Here's how the part is built. I have some questions about the finished solid (model axes, mm). A direction names the side the tool comes from. Round coordinates to 2 decimals unless told otherwise and drop trailing zeros. Loops run counter-clockwise (first coordinate to the right, second up) from the corner with the lowest first, then second, coordinate; pieces in that order, holes last. Notation, with made-up numbers: (43, 44) -> (94, 44) arc R30 ccw to (94, 66) -> close; hole circle Ø5 at (-29, 68). An arc over 180 degrees is marked (long way). Use CSV: the item, a comma, the result in double quotes. Start each with the question number.
from build123d import *

# Parameters (mm, degrees)
ESTRUSIONE_ESTRUSIONE1_DEPTH           = 5
SCHIZZO2_W                             = 20
SCHIZZO2_H                             = 6
TAGLIO_ESTRUSIONE1_DEPTH               = 4
FORO_SVASATO_PER_VITE_M2_1_D           = 2.4
FORO_SVASATO_PER_VITE_M2_1_DEPTH       = 4
FORO_SVASATO_PER_VITE_M2_1_CSINK_D     = 4.4
FORO_SVASATO_PER_VITE_M2_1_CSINK_ANGLE = 90
SCHIZZO6_R                             = 2
TAGLIO_ESTRUSIONE3_DEPTH               = 38
SCHIZZO8_R                             = 3
TAGLIO_ESTRUSIONE4_DEPTH               = 3
FORO_SVASATO_PER_VITE_M2_2_D           = 2.4
FORO_SVASATO_PER_VITE_M2_2_DEPTH       = 4
FORO_SVASATO_PER_VITE_M2_2_CSINK_D     = 4.4
FORO_SVASATO_PER_VITE_M2_2_CSINK_ANGLE = 90


with BuildPart() as part:
    # Schizzo1 → Estrusione-Estrusione1 (new body)
    with BuildSketch(Plane(origin=(0, 0, 0), x_dir=(1, 0, 0), z_dir=(0, 1, 0))):
        with BuildLine():
            Line((-29.167003354, 45), (90.832996646, 45))
            Line((90.832996646, 45), (110.832996646, 25))
            Line((110.832996646, 25), (110.832996646, -25))
            Line((110.832996646, -25), (90.832996646, -45))
            Line((90.832996646, -45), (-29.167003354, -45))
            ThreePointArc((-29.167003354, -45), (-36.238071166, -42.071067812), (-39.167003354, -35))
            Line((-39.167003354, -35), (-39.167003354, 35))
            ThreePointArc((-39.167003354, 35), (-36.238071166, 42.071067812), (-29.167003354, 45))
        make_face()
    extrude(amount=ESTRUSIONE_ESTRUSIONE1_DEPTH)

    # Schizzo2 → Taglio-Estrusione1 (cut)
    with BuildSketch(Plane.XZ):
        with Locations((20.832996646, -32)):
            Rectangle(SCHIZZO2_W, SCHIZZO2_H)
    extrude(amount=-TAGLIO_ESTRUSIONE1_DEPTH, mode=Mode.SUBTRACT)

    # Foro svasato per Vite M2-1
    with Locations(Plane(origin=(0, 4, 0), x_dir=(-1, 0, 0), z_dir=(0, -1, 0))):
        with Locations((-15.832996646, 32), (-25.832996646, 32)):
            CounterSinkHole(FORO_SVASATO_PER_VITE_M2_1_D / 2, FORO_SVASATO_PER_VITE_M2_1_CSINK_D / 2, depth=FORO_SVASATO_PER_VITE_M2_1_DEPTH, counter_sink_angle=FORO_SVASATO_PER_VITE_M2_1_CSINK_ANGLE)

    # Schizzo6 → Taglio-Estrusione3 (cut)
    with BuildSketch(Plane.XZ):
        with Locations(Location((-9.377003354, 22, 0), (0, 0, 270))):
            Circle(SCHIZZO6_R)
        with Locations(Location((72.302996646, 22, 0), (0, 0, 270))):
            Circle(SCHIZZO6_R)
        with Locations(Location((72.302996646, -22, 0), (0, 0, 270))):
            Circle(SCHIZZO6_R)
        with Locations(Location((-9.377003354, -22, 0), (0, 0, 270))):
            Circle(SCHIZZO6_R)
    extrude(amount=-TAGLIO_ESTRUSIONE3_DEPTH, mode=Mode.SUBTRACT)

    # Schizzo8 → Taglio-Estrusione4 (cut)
    with BuildSketch(Plane.XZ):
        with Locations(Location((-31.167003354, 40, 0), (0, 0, 270))):
            Circle(SCHIZZO8_R)
        with Locations(Location((30.832996646, 41.5, 0), (0, 0, 270))):
            Circle(SCHIZZO8_R)
        with Locations(Location((97.347715272, 30, 0), (0, 0, 270))):
            Circle(SCHIZZO8_R)
        with Locations(Location((97.347715272, -30, 0), (0, 0, 270))):
            Circle(SCHIZZO8_R)
        with Locations(Location((30.832996646, -41.5, 0), (0, 0, 270))):
            Circle(SCHIZZO8_R)
        with Locations(Location((-31.167003354, -40, 0), (0, 0, 270))):
            Circle(SCHIZZO8_R)
    extrude(amount=-TAGLIO_ESTRUSIONE4_DEPTH, mode=Mode.SUBTRACT)

    # Foro svasato per Vite M2-2
    with Locations(Plane(origin=(0, 3, 0), x_dir=(-1, 0, 0), z_dir=(0, -1, 0))):
        with Locations((31.161216293, -39.892156873), (-30.832996646, -41.5), (-97.347715272, -30), (-97.347715272, 30), (-30.832996646, 41.5), (31.167003354, 40)):
            CounterSinkHole(FORO_SVASATO_PER_VITE_M2_2_D / 2, FORO_SVASATO_PER_VITE_M2_2_CSINK_D / 2, depth=FORO_SVASATO_PER_VITE_M2_2_DEPTH, counter_sink_angle=FORO_SVASATO_PER_VITE_M2_2_CSINK_ANGLE)


solid = part.part
Q1. I need wall thicknesses on line 1 along Z through (x, y) = (72.5, 4.15); line 2 along X through (y, z) = (3.25, -22); line 3 along Z through (x, y) = (33.5, 2.7). Which ranges of each line are inside material? Lowest first, please.
Q2. I want a section at A-A, the plane z = 22. List the corners of the cut face in (x, y) for me.
Q3. For faces 1 (the flat face through (21, 2, -29)), 2 (the flat face through (100.973, 2.465, 34.86)), which set-ups out of +Z, -Z, +X, -X, +Y, -Y let a thin tool reach every point of the face, with its end or its side?
Q4. Will these pins go through, and if not, where does the flat tip stop? pin 1 Ø3 at (x, z) = (30.83, 41.5) entering from -Y; pin 2 Ø1.8 at (x, z) = (97.5, 28.5) entering from -Y; pin 3 Ø3 at (y, z) = (2.5, -31) entering from +X.
Q5. If we mould it in two halves opening along X, with no side actions, what happens to faces 3 (the flat face through (99, 3, -28)), 4 (the flat face through (37, 5, -1)), 5 (the flat face through (-39.167, 2, 0)), 6 (the flat face through (30.833, 2, -32))? For each: pulls with the +X half, pulls with the -X half, needs draft (parallel to the pull), parting line crosses it, or undercut.
Values found:
1,line 1,"-45 to -23.99, -20.01 to 20.01, 23.99 to 45"
1,line 2,"-39.17 to -11.38, -7.38 to 70.3, 74.3 to 110.83"
1,line 3,"-45 to -42.87, -40.13 to 40.13, 42.87 to 45"
2,outline,"(-39.17, 0) -> (-11.38, 0) -> (-11.38, 5) -> (-39.17, 5) -> close; (-7.38, 0) -> (70.3, 0) -> (70.3, 5) -> (-7.38, 5) -> close; (74.3, 0) -> (110.83, 0) -> (110.83, 5) -> (74.3, 5) -> close"
3,face 1,"-Y"
3,face 2,"+Z, +X, +Y, -Y"
4,pin 1,"y = 3.7"
4,pin 2,"y = 3"
4,pin 3,"x = 106.33"
5,face 3,"undercut"
5,face 4,"needs draft"
5,face 5,"pulls with the -X half"
5,face 6,"undercut"
